```python
from build123d import *

# Parameters (mm, degrees)
SKETCH1_W           = 63.5
SKETCH1_H           = 254
BOSS_EXTRUDE1_DEPTH = 3.175
SKETCH4_R           = 13.335
BOSS_EXTRUDE4_DEPTH = 3.175
SKETCH5_R           = 2.5
MOTOR_HOLES_DEPTH   = 245.142429639
SKETCH7_R           = 2.159
CUT_EXTRUDE2_DEPTH  = 245.142429639
FILLET1_R           = 12.7
FILLET2_R           = 6.35


with BuildPart() as part:
    # Sketch1 → Boss-Extrude1 (new body)
    with BuildSketch(Plane(origin=(0, 0, 0), x_dir=(1, 0, 0), z_dir=(0, 1, 0))):
        Polygon((-44.45, 139.7), (44.45, 139.7), (184.15, 139.7), (184.15, 120.65), (44.45, 120.65), (44.45, -120.65), (184.15, -120.65), (184.15, -139.7), (44.45, -139.7), (-44.45, -139.7), (-184.15, -139.7), (-184.15, -120.65), (-44.45, -120.65), (-44.45, 120.65), (-184.15, 120.65), (-184.15, 139.7), align=None)
        Rectangle(SKETCH1_W, SKETCH1_H, mode=Mode.SUBTRACT)
    extrude(amount=BOSS_EXTRUDE1_DEPTH)

    # Sketch4 → Boss-Extrude4 (add)
    with BuildSketch(Plane(origin=(0, 3.175, 0), x_dir=(1, 0, 0), z_dir=(0, 1, 0))):
        with Locations((184.15, 130.175)):
            Circle(SKETCH4_R)
        with Locations((-184.15, 130.175)):
            Circle(SKETCH4_R)
        with Locations((-184.15, -130.175)):
            Circle(SKETCH4_R)
        with Locations((184.15, -130.175)):
            Circle(SKETCH4_R)
    extrude(amount=-BOSS_EXTRUDE4_DEPTH)

    # Sketch5 → Motor Holes (cut, through all)
    with BuildSketch(Plane(origin=(0, 3.175, 0), x_dir=(1, 0, 0), z_dir=(0, 1, 0))):
        with Locations(Location((184.15, 130.175, 0), (0, 0, 270))):
            Circle(SKETCH5_R)
        with Locations(Location((-184.15, 130.175, 0), (0, 0, 90))):
            Circle(SKETCH5_R)
        with Locations(Location((184.15, -130.175, 0), (0, 0, 90))):
            Circle(SKETCH5_R)
        with Locations(Location((-184.15, -130.175, 0), (0, 0, 270))):
            Circle(SKETCH5_R)
        with BuildLine():
            Line((173.650002, 131.425), (175.649998, 131.425))
            ThreePointArc((175.649998, 131.425), (176.899998, 130.175), (175.649998, 128.925))
            Line((175.649998, 128.925), (173.650002, 128.925))
            ThreePointArc((173.650002, 128.925), (172.400002, 130.175), (173.650002, 131.425))
        make_face()
        with BuildLine():
            Line((194.649998, 131.425), (192.650002, 131.425))
            ThreePointArc((192.650002, 131.425), (191.400002, 130.175), (192.650002, 128.925))
            Line((192.650002, 128.925), (194.649998, 128.925))
            ThreePointArc((194.649998, 128.925), (195.899998, 130.175), (194.649998, 131.425))
        make_face()
        with BuildLine():
            Line((185.4, 139.175), (185.4, 137.175))
            ThreePointArc((185.4, 137.175), (184.15, 135.925), (182.9, 137.175))
            Line((182.9, 137.175), (182.9, 139.175))
            ThreePointArc((182.9, 139.175), (184.15, 140.425), (185.4, 139.175))
        make_face()
        with BuildLine():
            Line((185.4, 121.175), (185.4, 123.175))
            ThreePointArc((185.4, 123.175), (184.15, 124.425), (182.9, 123.175))
            Line((182.9, 123.175), (182.9, 121.175))
            ThreePointArc((182.9, 121.175), (184.15, 119.925), (185.4, 121.175))
        make_face()
        with BuildLine():
            Line((-173.650002, 131.425), (-175.649998, 131.425))
            ThreePointArc((-175.649998, 131.425), (-176.899998, 130.175), (-175.649998, 128.925))
            Line((-175.649998, 128.925), (-173.650002, 128.925))
            ThreePointArc((-173.650002, 128.925), (-172.400002, 130.175), (-173.650002, 131.425))
        make_face()
        with BuildLine():
            Line((-194.649998, 131.425), (-192.650002, 131.425))
            ThreePointArc((-192.650002, 131.425), (-191.400002, 130.175), (-192.650002, 128.925))
            Line((-192.650002, 128.925), (-194.649998, 128.925))
            ThreePointArc((-194.649998, 128.925), (-195.899998, 130.175), (-194.649998, 131.425))
        make_face()
        with BuildLine():
            Line((-185.4, 139.175), (-185.4, 137.175))
            ThreePointArc((-185.4, 137.175), (-184.15, 135.925), (-182.9, 137.175))
            Line((-182.9, 137.175), (-182.9, 139.175))
            ThreePointArc((-182.9, 139.175), (-184.15, 140.425), (-185.4, 139.175))
        make_face()
        with BuildLine():
            Line((-185.4, 121.175), (-185.4, 123.175))
            ThreePointArc((-185.4, 123.175), (-184.15, 124.425), (-182.9, 123.175))
            Line((-182.9, 123.175), (-182.9, 121.175))
            ThreePointArc((-182.9, 121.175), (-184.15, 119.925), (-185.4, 121.175))
        make_face()
        with BuildLine():
            Line((173.650002, -131.425), (175.649998, -131.425))
            ThreePointArc((175.649998, -131.425), (176.899998, -130.175), (175.649998, -128.925))
            Line((175.649998, -128.925), (173.650002, -128.925))
            ThreePointArc((173.650002, -128.925), (172.400002, -130.175), (173.650002, -131.425))
        make_face()
        with BuildLine():
            Line((185.4, -139.175), (185.4, -137.175))
            ThreePointArc((185.4, -137.175), (184.15, -135.925), (182.9, -137.175))
            Line((182.9, -137.175), (182.9, -139.175))
            ThreePointArc((182.9, -139.175), (184.15, -140.425), (185.4, -139.175))
        make_face()
        with BuildLine():
            Line((194.649998, -131.425), (192.650002, -131.425))
            ThreePointArc((192.650002, -131.425), (191.400002, -130.175), (192.650002, -128.925))
            Line((192.650002, -128.925), (194.649998, -128.925))
            ThreePointArc((194.649998, -128.925), (195.899998, -130.175), (194.649998, -131.425))
        make_face()
        with BuildLine():
            Line((185.4, -121.175), (185.4, -123.175))
            ThreePointArc((185.4, -123.175), (184.15, -124.425), (182.9, -123.175))
            Line((182.9, -123.175), (182.9, -121.175))
            ThreePointArc((182.9, -121.175), (184.15, -119.925), (185.4, -121.175))
        make_face()
        with BuildLine():
            Line((-185.4, -121.175), (-185.4, -123.175))
            ThreePointArc((-185.4, -123.175), (-184.15, -124.425), (-182.9, -123.175))
            Line((-182.9, -123.175), (-182.9, -121.175))
            ThreePointArc((-182.9, -121.175), (-184.15, -119.925), (-185.4, -121.175))
        make_face()
        with BuildLine():
            Line((-185.4, -139.175), (-185.4, -137.175))
            ThreePointArc((-185.4, -137.175), (-184.15, -135.925), (-182.9, -137.175))
            Line((-182.9, -137.175), (-182.9, -139.175))
            ThreePointArc((-182.9, -139.175), (-184.15, -140.425), (-185.4, -139.175))
        make_face()
        with BuildLine():
            Line((-194.649998, -131.425), (-192.650002, -131.425))
            ThreePointArc((-192.650002, -131.425), (-191.400002, -130.175), (-192.650002, -128.925))
            Line((-192.650002, -128.925), (-194.649998, -128.925))
            ThreePointArc((-194.649998, -128.925), (-195.899998, -130.175), (-194.649998, -131.425))
        make_face()
        with BuildLine():
            Line((-173.650002, -131.425), (-175.649998, -131.425))
            ThreePointArc((-175.649998, -131.425), (-176.899998, -130.175), (-175.649998, -128.925))
            Line((-175.649998, -128.925), (-173.650002, -128.925))
            ThreePointArc((-173.650002, -128.925), (-172.400002, -130.175), (-173.650002, -131.425))
        make_face()
    extrude(amount=-MOTOR_HOLES_DEPTH, mode=Mode.SUBTRACT)

    # Sketch7 → Cut-Extrude2 (cut, through all)
    with BuildSketch(Plane(origin=(0, 3.175, 0), x_dir=(1, 0, 0), z_dir=(0, 1, 0))):
        with Locations(Location((-38.1, 133.35, 0), (0, 0, 270))):
            Circle(SKETCH7_R)
        with Locations(Location((-38.1, 66.675, 0), (0, 0, 270))):
            Circle(SKETCH7_R)
        with Locations(Location((-38.1, 0, 0), (0, 0, 270))):
            Circle(SKETCH7_R)
        with Locations(Location((-38.1, -66.675, 0), (0, 0, 270))):
            Circle(SKETCH7_R)
        with Locations(Location((-38.1, -133.35, 0), (0, 0, 270))):
            Circle(SKETCH7_R)
        with Locations(Location((38.1, -133.35, 0), (0, 0, 90))):
            Circle(SKETCH7_R)
        with Locations(Location((38.1, -66.675, 0), (0, 0, 90))):
            Circle(SKETCH7_R)
        with Locations(Location((38.1, 0, 0), (0, 0, 90))):
            Circle(SKETCH7_R)
        with Locations(Location((38.1, 66.675, 0), (0, 0, 90))):
            Circle(SKETCH7_R)
        with Locations(Location((38.1, 133.35, 0), (0, 0, 90))):
            Circle(SKETCH7_R)
        with Locations(Location((0, 133.35, 0), (0, 0, 270))):
            Circle(SKETCH7_R)
        with Locations(Location((0, -133.35, 0), (0, 0, 90))):
            Circle(SKETCH7_R)
    extrude(amount=-CUT_EXTRUDE2_DEPTH, mode=Mode.SUBTRACT)

    # Fillet1
    fillet1_edges = [part.edges().sort_by_distance(p)[0] for p in [
        (-31.75, 1.5875, -127),
        (-31.75, 1.5875, 127),
        (31.75, 1.5875, 127),
        (31.75, 1.5875, -127),
    ]]
    fillet(fillet1_edges, radius=FILLET1_R)

    # Fillet2
    fillet2_edges = [part.edges().sort_by_distance(p)[0] for p in [
        (44.45, 1.5875, -120.65),
        (44.45, 1.5875, 120.65),
        (-44.45, 1.5875, 120.65),
        (-44.45, 1.5875, -120.65),
    ]]
    fillet(fillet2_edges, radius=FILLET2_R)


solid = part.part
```
CAD build for the part. Positions are in the model's coordinates, mm. A direction names the side the tool comes from. Coordinates: 2 decimals unless noted, no trailing zeros. Order: outer loops, then holes, each group sorted by start corner. A loop starts at its lowest first (then second) coordinate and runs counter-clockwise, first axis right, second up. Notation, with made-up numbers: (36.5, 65) - (64.5, 65) arc R15 ccw to (64.5, 75) - close; hole circle Ø2 at (-2, 84). An arc over 180 degrees is marked (long way). Answer in a Markdown table with one row per item.
1. Slice it at B-B, the plane z = -7. List the corners of the cut face in (x, y) (3 decimals).
Answer:
| item | result |
|---|---|
| outline | (-44.45, 0) - (-31.75, 0) - (-31.75, 3.175) - (-44.45, 3.175) - close; (31.75, 0) - (44.45, 0) - (44.45, 3.175) - (31.75, 3.175) - close |
2. Slice it at A-A, the plane x = 127.5. List the corners of the cut face in (y, z) (3 decimals).
Answer:
| item | result |
|---|---|
| outline | (0, -139.7) - (3.175, -139.7) - (3.175, -120.65) - (0, -120.65) - close; (0, 120.65) - (3.175, 120.65) - (3.175, 139.7) - (0, 139.7) - close |
3. Slice it at C-C, the plane y = 2.4. Give the number of separate pieces and of enclosed holes in the cut face, then the cut area to 3 significant figures.
Answer:
| item | result |
|---|---|
| separate pieces | 1 |
| enclosed holes | 33 |
| area | 20,400 mm² |
4. Pull direction Z, two halves, no side cores. Call faces 1 (the face through (197.478, 1.61, -129.737)), 2 (the face through (28.13, 1.61, -123.18)), 3 (the face through (43, 0, -11)): +Z half, -Z half, draft (parallel to the pull), parting line (faces both ways), or undercut.
Answer:
| item | result |
|---|---|
| face 1 | undercut |
| face 2 | undercut |
| face 3 | draft |
5. Drill centre lines: L1, parallel to Z at x = 38.1, y = 2.05; L2, parallel to X at y = 1.8, z = -100. Where is each one in solid material? Low to high. Write a range as from..to.
Answer:
| item | result |
|---|---|
| L1 | -139.7..-135.51, -131.19..-68.83, -64.52..-2.16, 2.16..64.52, 68.83..131.19, 135.51..139.7 |
| L2 | -44.45..-31.75, 31.75..44.45 |
6. 3-axis set-ups, long thin cutter, end or side, ignore diameter. For faces 4 (the face through (43, 3.175, -11)), 5 (the face through (28.13, 1.61, 123.18)): which of +Z, -Z, +X, -X, +Y, -Y reach the whole face in a straight line?
Answer:
| item | result |
|---|---|
| face 4 | +Z, -Z, +X, -X, +Y |
| face 5 | +Y, -Y |
7. Flat gauge pins, fed straight in: P1, Ø1, axis at x = 34, z = 66, coming from the -Y side; P2, Ø1, axis at x = 193.5, y = 1.5, coming from the -Z side; P3, Ø1.6, axis at y = 1, z = 25, coming from the +X side; P4, Ø4, axis at x = -38.1, z = 0, coming from the +Y side. Where does each tip first touch, or does it go through?
Answer:
| item | result |
|---|---|
| P1 | y = 0 |
| P2 | z = -140.15 |
| P3 | x = 44.45 |
| P4 | through |
